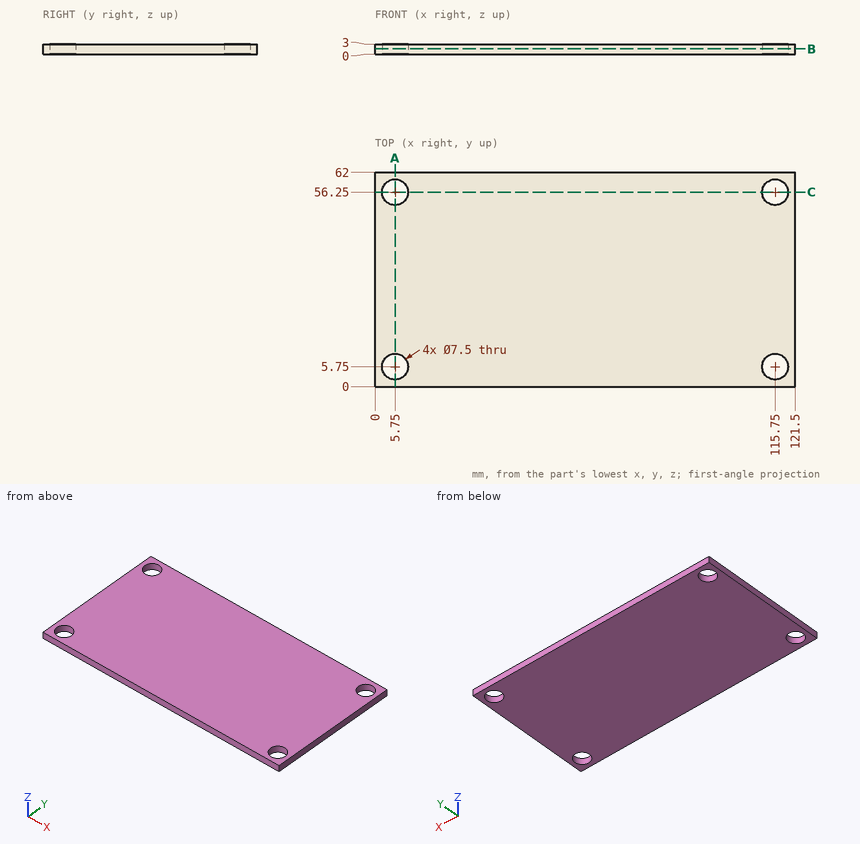
Design review of the part shown in the three views and the two pictorial views. Dimensions are in mm from the part's minimum x, y and z. Round coordinates to 2 decimals unless told otherwise and drop trailing zeros. Write each loop counter-clockwise with the first axis right and the second up, starting at its lowest first coordinate (ties: lowest second). Pieces come first, ordered by that corner, then holes. Notation, with made-up numbers: (-6, 81.5) - (27, 81.5) arc R28 ccw to (27, 115.5) - close; hole circle Ø8 at (88.25, -1). An arc over 180 degrees is marked (long way). Write item = value, one per line. Start each with the question number.
1. Consider section A-A on x = 5.75. State the section outline as (y, z) points, plus the area to 3 significant figures.
2. Wall thickness on L1, parallel to Y at x = 5.75, z = 1.8; L2, parallel to X at y = 8.5, z = 0.8: over which ranges is each line inside the solid? List them lowest first.
3. Consider section B-B on z = 1.6. State the section outline as (x, y) points.
4. Consider section C-C on y = 56.25. State the section outline as (x, z) points.
Evaluation:
q1.outline = (0, 0) - (2, 0) - (2, 3) - (0, 3) - close; (9.5, 0) - (52.5, 0) - (52.5, 3) - (9.5, 3) - close; (60, 0) - (62, 0) - (62, 3) - (60, 3) - close
q1.area = 141 mm2
q2.L1 = 0 to 2, 9.5 to 52.5, 60 to 62
q2.L2 = 0 to 3.2, 8.3 to 113.2, 118.3 to 121.5
q3.outline = (0, 0) - (121.5, 0) - (121.5, 62) - (0, 62) - close; hole circle Ø7.5 at (5.75, 5.75); hole circle Ø7.5 at (5.75, 56.25); hole circle Ø7.5 at (115.75, 5.75); hole circle Ø7.5 at (115.75, 56.25)
q4.outline = (0, 0) - (2, 0) - (2, 3) - (0, 3) - close; (9.5, 0) - (112, 0) - (112, 3) - (9.5, 3) - close; (119.5, 0) - (121.5, 0) - (121.5, 3) - (119.5, 3) - close
